Geometry: final body of the model. Coordinates: model frame, mm. Face numbers are marked on the shaded views. A direction names the side the tool comes from. Give positions to 0.01 mm unless a question says otherwise; leave off trailing zeros. Order: outer loops, then holes, each group sorted by start corner. A loop starts at its lowest first (then second) coordinate and runs counter-clockwise, first axis right, second up. Notation, with made-up numbers: (65.25, 44.5) - (82.25, 44.5) arc R22 cw to (82.25, 67.5) - close; hole circle Ø5 at (61, 2.5). An arc over 180 degrees is marked (long way). Write item = value, one per line. Start each with the question number.
from build123d import *

# Parameters (mm, degrees)
SKIZZE1_R                       = 2.5
AUFSATZ_LINEAR_AUSTRAGEN1_DEPTH = 3.4
SKIZZE2_R                       = 3.5
AUFSATZ_LINEAR_AUSTRAGEN2_DEPTH = 1
SKIZZE3_R                       = 5
AUFSATZ_LINEAR_AUSTRAGEN3_DEPTH = 1


with BuildPart() as part:
    # Skizze1 → Aufsatz-Linear austragen1 (new body)
    with BuildSketch(Plane.XY):
        Circle(SKIZZE1_R)
    extrude(amount=-AUFSATZ_LINEAR_AUSTRAGEN1_DEPTH)

    # Skizze2 → Aufsatz-Linear austragen2 (add)
    with BuildSketch(Plane(origin=(0, 0, -3.4), x_dir=(-1, 0, 0), z_dir=(0, 0, -1))):
        Circle(SKIZZE2_R)
    extrude(amount=AUFSATZ_LINEAR_AUSTRAGEN2_DEPTH)

    # Skizze3 → Aufsatz-Linear austragen3 (add)
    with BuildSketch(Plane.XY):
        Circle(SKIZZE3_R)
    extrude(amount=AUFSATZ_LINEAR_AUSTRAGEN3_DEPTH)


solid = part.part
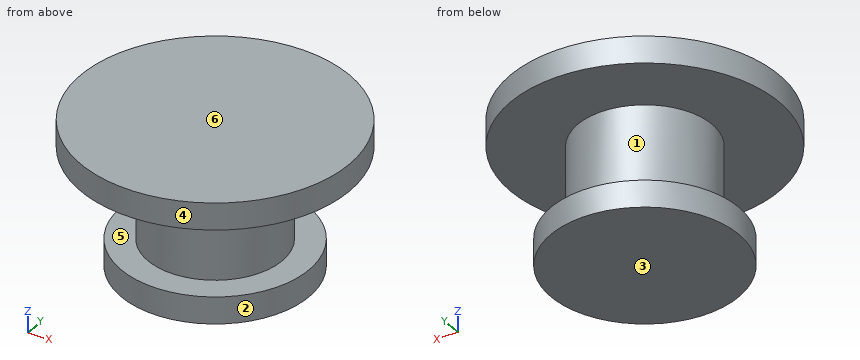
Q1. Contact query for a flat-ended pin moving along its axis: pin 1 (2 mm diameter, centred on x = -4, z = -0.5, fed in from +Y). Output: stop coordinate, or through.
Q2. Section D-D, the plane z = -1.4. Return the cut outline in (x, y).
Q3. Section C-C, the plane x = -3. Return the cut outline in (y, z), then the cut area to 3 significant figures.
Q4. Material intervals for line 1 along Z through (x, y) = (-2.5, 2.25); line 2 along Z through (x, y) = (-4.25, -2.5); line 3 along X through (y, z) = (-1, -2.8), sorted ascending. Write a range as from..to.
Q5. Pull-direction query (Z, two-part tool) for the marked faces 3, 4, 5 and 6; classes: +Z half, -Z half, draft (parallel to the pull), parting line (faces both ways), or undercut.
Q6. Section A-A, the plane y = 0. Return the cut outline in (x, z).
Q7. Set-up query: the marked faces 1 and 2. Return all of +Z, -Z, +X, -X, +Y, -Y with unobstructed straight access to the full face (end or side cutting, diameter ignored); none if empty.
The answers:
q1.pin_1 = 3.9
q2.outline = circle Ø5 at (0, 0)
q3.outline = (-4, 0) - (4, 0) - (4, 1) - (-4, 1) - close; (-1.8, -4.4) - (1.8, -4.4) - (1.8, -3.4) - (-1.8, -3.4) - close
q3.area = 11.6 mm²
q4.line_1 = -4.4..-3.4, 0..1
q4.line_2 = 0..1
q4.line_3 = -2.29..2.29
q5.face_3 = -Z half
q5.face_4 = draft
q5.face_5 = undercut
q5.face_6 = +Z half
q6.outline = (-5, 0) - (-2.5, 0) - (-2.5, -3.4) - (-3.5, -3.4) - (-3.5, -4.4) - (3.5, -4.4) - (3.5, -3.4) - (2.5, -3.4) - (2.5, 0) - (5, 0) - (5, 1) - (-5, 1) - close
q7.face_1 = none
q7.face_2 = -Z
